Answer from the drawing. Dimensions are ordinates in mm from the lowest x, y and z of the part. Coordinates: 2 decimals unless noted, no trailing zeros. Write each loop counter-clockwise with the first axis right and the second up, starting at its lowest first coordinate (ties: lowest second). Pieces come first, ordered by that corner, then holes. Notation, with made-up numbers: (45.25, 18.25) -> (57.25, 18.25) arc R24 cw to (57.25, 54.25) -> close; hole circle Ø10 at (87, -39). An arc over 180 degrees is marked (long way). One line per item, written item: value. Start each with the question number.
1. For a pull along Z with two mould halves and no side action, classify the marked faces 1, 2 and 3 as pulls with the +Z half, pulls with the -Z half, needs draft (parallel to the pull), parting line crosses it, or undercut.
2. Find section C-C, the plane y = 75.5. Write down the section's boundary in (x, z) (1 decimal), and give its area (3 significant figures).
3. Find section B-B, the plane x = 32. Write down the section's boundary in (y, z) (1 decimal), and give its area (3 significant figures).
4. Find section D-D, the plane z = 54. Write down the section's boundary in (x, y).
5. Consider line 1 along Z through (x, y) = (24, 63.5) (1 decimal); line 2 along Z through (x, y) = (92, 82.5); line 3 along Y through (x, z) = (87.5, 32.5) (1 decimal). Determine where each line is inside the solid, lowest interval first.
6. Find section A-A, the plane z = 71. Write down the section's boundary in (x, y).
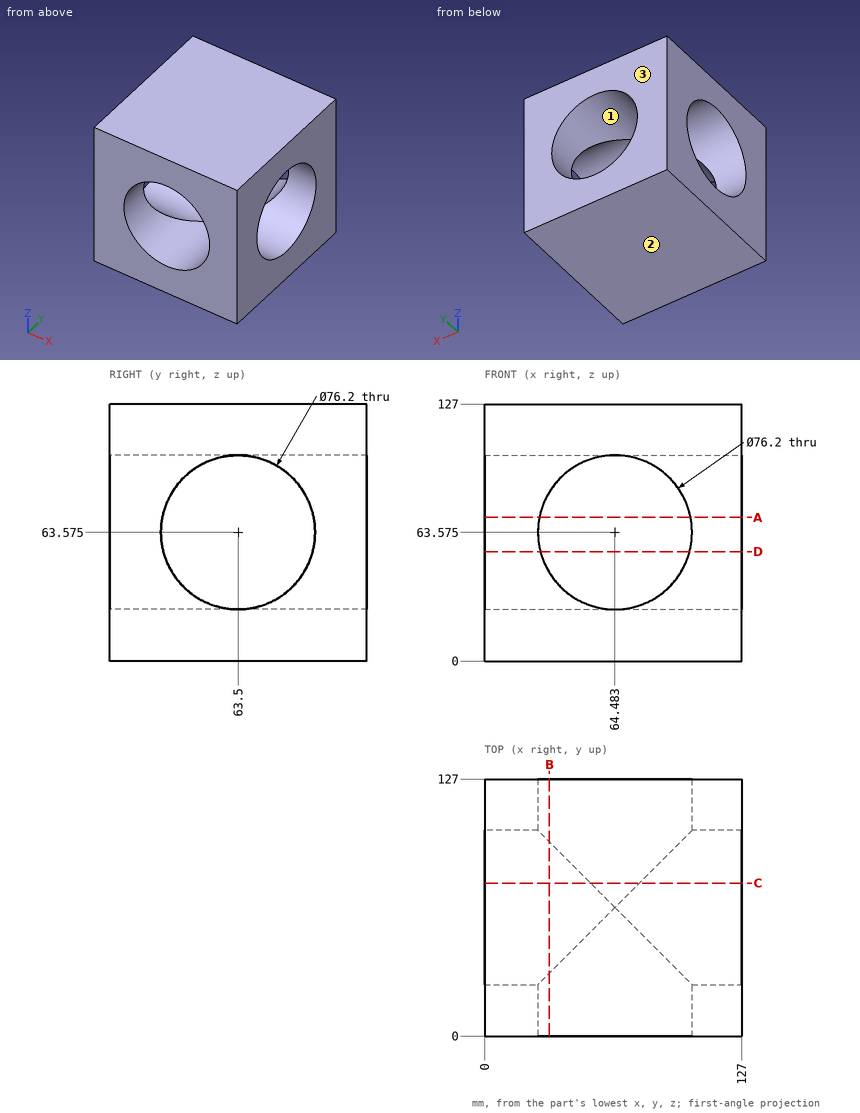
Answer block:
1. face 1: undercut
1. face 2: pulls with the -Z half
1. face 3: needs draft
2. outline: (0, 0) -> (127, 0) -> (127, 27.4) -> (76.5, 27.4) arc R38.1 cw to (52.5, 27.4) -> (0, 27.4) -> close; (0, 99.7) -> (52.5, 99.7) arc R38.1 cw to (76.5, 99.7) -> (127, 99.7) -> (127, 127) -> (0, 127) -> close
2. area: 6,880 mm2
3. outline: (0, 0) -> (127, 0) -> (127, 43.7) -> (96, 43.7) arc R38.1 cw to (31, 43.7) -> (0, 43.7) -> close; (0, 83.5) -> (31, 83.5) arc R38.1 cw to (96, 83.5) -> (127, 83.5) -> (127, 127) -> (0, 127) -> close
3. area: 9,400 mm2
4. outline: (0, 0) -> (27.61, 0) -> (27.61, 26.62) -> (0, 26.62) -> close; (0, 100.38) -> (27.61, 100.38) -> (27.61, 127) -> (0, 127) -> close; (101.36, 0) -> (127, 0) -> (127, 26.62) -> (101.36, 26.62) -> close; (101.36, 100.38) -> (127, 100.38) -> (127, 127) -> (101.36, 127) -> close
5. line 1: z = 0 to 25.5, 101.7 to 127
5. line 2: z = 0 to 30.55, 96.6 to 127
5. line 3: y = 0 to 41.5, 85.5 to 127
6. outline: (0, 0) -> (27.11, 0) -> (27.11, 26.13) -> (0, 26.13) -> close; (0, 100.87) -> (27.11, 100.87) -> (27.11, 127) -> (0, 127) -> close; (101.85, 0) -> (127, 0) -> (127, 26.13) -> (101.85, 26.13) -> close; (101.85, 100.87) -> (127, 100.87) -> (127, 127) -> (101.85, 127) -> close
